Input: part model. Units: mm. Frame: model coordinates. A direction names the side the tool comes from. Round coordinates to 2 decimals unless told otherwise and drop trailing zeros. Write each loop counter-clockwise with the first axis right and the second up, starting at its lowest first coordinate (ties: lowest second). Pieces come first, ordered by that corner, then holes. Notation, with made-up numbers: M -18,-13 L -2,-13 A16 ccw -2,-8 Z; hole C 64.5,-25 d10. An arc over 180 degrees is marked long. Write each question's results on one line, items separated by ' | '. Start each with the question number.
```python
from build123d import *

# Parameters (mm, degrees)
SERVICE_BOW_DEPTH = 4


with BuildPart() as part:
    # 草图1 → Service_Bow (new body)
    with BuildSketch(Plane.XY):
        Polygon((0.238238251, -1.985759939), (6.052696728, -1.00199462), (11.851815581, 0.543134876), (17.629770487, 2.623716718), (23.383882437, 5.20057493), (29.113972134, 8.223185483), (34.821368817, 11.631260703), (40.508013578, 15.356118412), (46.175832601, 19.322053213), (51.826370472, 23.44786233), (57.46060541, 27.648580809), (63.078870472, 31.837413257), (68.680832601, 35.92781796), (74.265513578, 39.8356909), (79.831368817, 43.481597056), (85.376472134, 46.792990637), (90.898882437, 49.706339676), (96.397270487, 52.169010306), (101.871815581, 54.140678109), (107.325196728, 55.593980706), (112.763238251, 56.514240061), (118.194648786, 56.898458582), (123.629616677, 56.754246479), (129.077741493, 56.099396062), (134.546278673, 54.962260391), (140.039426657, 53.382396607), (145.558668032, 51.410746743), (151.103674368, 49.108979529), (156.673265064, 46.548051938), (162.266147999, 43.806258645), (167.881387728, 40.967036021), (173.518647999, 38.116707719), (179.178265064, 35.342287191), (184.861174368, 32.729407041), (190.568668032, 30.36041039), (196.301926657, 28.312591454), (202.061278673, 26.656495644), (207.845241493, 25.454102473), (213.649616677, 24.756703246), (219.467148786, 24.602483256), (225.288238251, 25.014240061), (224.811761749, 28.985759939), (219.380351214, 28.601541418), (213.945383323, 28.745753521), (208.497258507, 29.400603938), (203.028721327, 30.537739609), (197.535573343, 32.117603393), (192.016331968, 34.089253257), (186.471325632, 36.391020471), (180.901734936, 38.951948062), (175.308852001, 41.693741355), (169.693612272, 44.532963979), (164.056352001, 47.383292281), (158.396734936, 50.157712809), (152.713825632, 52.770592959), (147.006331968, 55.13958961), (141.273073343, 57.187408546), (135.513721327, 58.843504356), (129.729758507, 60.045897527), (123.925383323, 60.743296754), (118.107851214, 60.897516744), (112.286761749, 60.485759939), (106.472303272, 59.50199462), (100.673184419, 57.956865124), (94.895229513, 55.876283282), (89.141117563, 53.29942507), (83.411027866, 50.276814517), (77.703631183, 46.868739297), (72.016986422, 43.143881588), (66.349167399, 39.177946787), (60.698629528, 35.05213767), (55.06439459, 30.851419191), (49.446129528, 26.662586743), (43.844167399, 22.57218204), (38.259486422, 18.6643091), (32.693631183, 15.018402944), (27.148527866, 11.707009363), (21.626117563, 8.793660324), (16.127729513, 6.330989694), (10.653184419, 4.359321891), (5.199803272, 2.906019294), (-0.238238251, 1.985759939), align=None)
    extrude(amount=SERVICE_BOW_DEPTH)


solid = part.part
```
1. Draft query along X for faces 1 (the face through (137.254, 54.183, 1.972)), 2 (the face through (104, 55, 0)), 3 (the face through (20.467, 3.894, 1.972)), 4 (the face through (2.519, 2.452, 1.972)). Return one class per face: +X half, -X half, draft (parallel to the pull), parting line (faces both ways), or undercut.
2. Line query: L1, parallel to Y at x = 198.5, z = 0.25; L2, parallel to X at y = 45, z = 2.7; L3, parallel to X at y = 44, z = 0.9. Output: solid intervals per line, ascending. Write a range as from..to.
3. Contact query for flat-ended pins moving along their axis: P1, Ø2, axis at y = 22, z = 2.5, coming from the +X side; P2, Ø8, axis at x = 130, y = 50.5, coming from the -Z side; P3, Ø1.5, axis at x = 199, z = 2.5, coming from the +Y side. Output: stop coordinate, or through.
4. Cut plane A-A on x = 104.5. Output: boundary loops of the cut face in (y, z).
5. Access query for faces 5 (the face through (69.223, 41.189, 1.972)), 6 (the face through (187.675, 31.561, 1.972)). Directions: +Z, -Z, +X, -X, +Y, -Y. A direction counts if a zero-diameter tool reaches every point of the face in a straight line with its end or side. Return the directions, or none.
Answers follow:
1) face 1: undercut | face 2: draft | face 3: +X half | face 4: -X half
2) L1: y = 27.68..31.84 | L2: x = 74.85..82.37, 159.83..168.77 | L3: x = 73.32..80.7, 161.87..170.75
3) P1: stops at x = 51.21 | P2: passes through | P3: stops at y = 31.91
4) outline: M 54.84,0 L 58.98,0 L 58.98,4 L 54.84,4 Z
5) face 5: +Z, -Z, -X, +Y | face 6: +Z, -Z, -Y
